from build123d import *

# Parameters (mm, degrees)
F1_DEPTH = 25.4
F0_R     = 4.1207252188
F2_DEPTH = 1.524
F4_DEPTH = 5.08
F5_R     = 4.826
F6_DEPTH = 7.62
F8_R     = 5.2675515525
F9_DEPTH = 12.7
F9_TAPER = -3


with BuildPart() as f1:
    # F0 (on Top) → F1 (new body, symmetric)
    with BuildSketch(Plane.XY):
        with BuildLine():
            ThreePointArc((1.0998522687, -0.6349999897), (1.2267258009, -0.3287001815), (1.27, 0))
            ThreePointArc((1.27, 0), (1.2267257989, 0.328700189), (1.0998522611, 0.635000003))
            ThreePointArc((1.0998522611, 0.635000003), (0.6349999985, 1.0998522637), (0, 1.27))
            ThreePointArc((0, 1.27), (-0.6349999991, 1.0998522633), (-1.0998522618, 0.6350000018))
            ThreePointArc((-1.0998522618, 0.6350000018), (-1.27, 3.4e-09), (-1.0998522652, -0.6349999959))
            ThreePointArc((-1.0998522652, -0.6349999959), (-0.6350000021, -1.0998522616), (0, -1.27))
            ThreePointArc((0, -1.27), (0.6350000051, -1.0998522598), (1.0998522687, -0.6349999897))
        make_face()
        with BuildLine():
            ThreePointArc((-1.0998522618, 0.6350000018), (-0.6349999991, 1.0998522633), (0, 1.27))
            ThreePointArc((0, 1.27), (-0.6350000007, 1.4401477376), (-1.0998522636, 1.9050000014))
            ThreePointArc((-1.0998522636, 1.9050000014), (-0.9729787264, 1.5987001881), (-0.9297045256, 1.27))
            ThreePointArc((-0.9297045256, 1.27), (-0.972978726, 0.9412998137), (-1.0998522618, 0.6350000018))
        make_face()
        with BuildLine():
            ThreePointArc((0, 1.27), (0.6349999985, 1.0998522637), (1.0998522611, 0.635000003))
            ThreePointArc((1.0998522611, 0.635000003), (0.9297045256, 1.2699999943), (1.0998522553, 1.904999987))
            ThreePointArc((1.0998522553, 1.904999987), (0.6349999935, 1.4401477334), (0, 1.27))
        make_face()
        with BuildLine():
            ThreePointArc((1.0998522611, 0.635000003), (1.2267257989, 0.328700189), (1.27, 0))
            ThreePointArc((1.27, 0), (1.2267258009, -0.3287001815), (1.0998522687, -0.6349999897))
            ThreePointArc((1.0998522687, -0.6349999897), (1.5647045337, -0.1701477325), (2.1997045323, 0))
            ThreePointArc((2.1997045323, 0), (1.564704527, 0.1701477364), (1.0998522611, 0.635000003))
        make_face()
        with BuildLine():
            ThreePointArc((1.0998522687, -1.9050000103), (0.9297045256, -1.27), (1.0998522687, -0.6349999897))
            ThreePointArc((1.0998522687, -0.6349999897), (0.6350000051, -1.0998522598), (0, -1.27))
            ThreePointArc((0, -1.27), (0.6350000051, -1.4401477402), (1.0998522687, -1.9050000103))
        make_face()
        with BuildLine():
            ThreePointArc((-1.0998522652, -1.9050000041), (-0.635000002, -1.4401477384), (0, -1.27))
            ThreePointArc((0, -1.27), (-0.6350000021, -1.0998522616), (-1.0998522652, -0.6349999959))
            ThreePointArc((-1.0998522652, -0.6349999959), (-0.9729787268, -0.9412998104), (-0.9297045256, -1.27))
            ThreePointArc((-0.9297045256, -1.27), (-0.9729787268, -1.5987001896), (-1.0998522652, -1.9050000041))
        make_face()
        with BuildLine():
            ThreePointArc((-1.0998522652, -0.6349999959), (-1.27, 3.4e-09), (-1.0998522618, 0.6350000018))
            ThreePointArc((-1.0998522618, 0.6350000018), (-1.5647045247, 0.1701477377), (-2.1997045256, 0))
            ThreePointArc((-2.1997045256, 0), (-1.5647045277, -0.170147736), (-1.0998522652, -0.6349999959))
        make_face()
        with BuildLine():
            ThreePointArc((-1.0998522636, 1.9050000014), (-0.6350000007, 1.4401477376), (0, 1.27))
            ThreePointArc((0, 1.27), (0.6349999935, 1.4401477334), (1.0998522553, 1.904999987))
            ThreePointArc((1.0998522553, 1.904999987), (1.2267257974, 2.2112998055), (1.27, 2.54))
            ThreePointArc((1.27, 2.54), (0.8980256121, 3.4380256121), (0, 3.81))
            ThreePointArc((0, 3.81), (-1.0998522624, 3.1750000007), (-1.0998522636, 1.9050000014))
        make_face()
        with BuildLine():
            ThreePointArc((-2.1997045256, 0), (-1.5647045247, 0.1701477377), (-1.0998522618, 0.6350000018))
            ThreePointArc((-1.0998522618, 0.6350000018), (-0.972978726, 0.9412998137), (-0.9297045256, 1.27))
            ThreePointArc((-0.9297045256, 1.27), (-0.9729787264, 1.5987001881), (-1.0998522636, 1.9050000014))
            ThreePointArc((-1.0998522636, 1.9050000014), (-2.1997045238, 2.54), (-3.2995567858, 1.9050000045))
            ThreePointArc((-3.2995567858, 1.9050000045), (-3.2995567897, 0.6350000022), (-2.1997045256, 0))
        make_face()
        with BuildLine():
            ThreePointArc((-0.9297045256, -1.27), (-0.9729787268, -0.9412998104), (-1.0998522652, -0.6349999959))
            ThreePointArc((-1.0998522652, -0.6349999959), (-1.5647045277, -0.170147736), (-2.1997045256, 0))
            ThreePointArc((-2.1997045256, 0), (-3.2995568097, -0.6350000369), (-3.2995567458, -1.9050000739))
            ThreePointArc((-3.2995567458, -1.9050000739), (-2.1997044853, -2.54), (-1.0998522652, -1.9050000041))
            ThreePointArc((-1.0998522652, -1.9050000041), (-0.9729787268, -1.5987001896), (-0.9297045256, -1.27))
        make_face()
        with BuildLine():
            ThreePointArc((1.0998522687, -1.9050000103), (0.6350000051, -1.4401477402), (0, -1.27))
            ThreePointArc((0, -1.27), (-0.635000002, -1.4401477384), (-1.0998522652, -1.9050000041))
            ThreePointArc((-1.0998522652, -1.9050000041), (-1.0998522616, -3.175000002), (0, -3.81))
            ThreePointArc((0, -3.81), (0.8980256121, -3.4380256121), (1.27, -2.54))
            ThreePointArc((1.27, -2.54), (1.2267258009, -2.2112998185), (1.0998522687, -1.9050000103))
        make_face()
        with BuildLine():
            ThreePointArc((2.1997045323, 0), (1.5647045337, -0.1701477325), (1.0998522687, -0.6349999897))
            ThreePointArc((1.0998522687, -0.6349999897), (0.9297045256, -1.27), (1.0998522687, -1.9050000103))
            ThreePointArc((1.0998522687, -1.9050000103), (2.1997045101, -2.54), (3.299556767, -1.9050000371))
            ThreePointArc((3.299556767, -1.9050000371), (3.4264303195, -1.598700208), (3.4697045256, -1.27))
            ThreePointArc((3.4697045256, -1.27), (3.0977301401, -0.3719743903), (2.1997045323, 0))
        make_face()
        with BuildLine():
            ThreePointArc((1.0998522553, 1.904999987), (0.9297045256, 1.2699999943), (1.0998522611, 0.635000003))
            ThreePointArc((1.0998522611, 0.635000003), (1.564704527, 0.1701477364), (2.1997045323, 0))
            ThreePointArc((2.1997045323, 0), (3.0977301401, 0.3719743903), (3.4697045256, 1.27))
            ThreePointArc((3.4697045256, 1.27), (3.4264303195, 1.598700208), (3.299556767, 1.9050000371))
            ThreePointArc((3.299556767, 1.9050000371), (2.1997044967, 2.54), (1.0998522553, 1.904999987))
        make_face()
    extrude(amount=F1_DEPTH, both=True)

    # F0 (on Top) → F2 (join, symmetric)
    with BuildSketch(Plane.XY):
        Circle(F0_R)
        with BuildLine():
            ThreePointArc((0, 3.81), (1.9049999814, 3.2995567991), (3.299556767, 1.9050000371))
            ThreePointArc((3.299556767, 1.9050000371), (3.6801773926, 0.9861005825), (3.81, 0))
            ThreePointArc((3.81, 0), (3.6801773926, -0.9861005825), (3.299556767, -1.9050000371))
            ThreePointArc((3.299556767, -1.9050000371), (1.9049999814, -3.2995567991), (0, -3.81))
            ThreePointArc((0, -3.81), (-1.9049999631, -3.2995568097), (-3.2995567458, -1.9050000739))
            ThreePointArc((-3.2995567458, -1.9050000739), (-3.81, -4.01e-08), (-3.2995567858, 1.9050000045))
            ThreePointArc((-3.2995567858, 1.9050000045), (-1.9049999978, 3.2995567897), (0, 3.81))
        make_face(mode=Mode.SUBTRACT)
        with BuildLine():
            ThreePointArc((-3.2995567858, 1.9050000045), (-2.1997045238, 2.54), (-1.0998522636, 1.9050000014))
            ThreePointArc((-1.0998522636, 1.9050000014), (-1.0998522624, 3.1750000007), (0, 3.81))
            ThreePointArc((0, 3.81), (-1.9049999978, 3.2995567897), (-3.2995567858, 1.9050000045))
        make_face()
        with BuildLine():
            ThreePointArc((1.27, 2.54), (1.2267257974, 2.2112998055), (1.0998522553, 1.904999987))
            ThreePointArc((1.0998522553, 1.904999987), (2.1997044967, 2.54), (3.299556767, 1.9050000371))
            ThreePointArc((3.299556767, 1.9050000371), (1.9049999814, 3.2995567991), (0, 3.81))
            ThreePointArc((0, 3.81), (0.8980256121, 3.4380256121), (1.27, 2.54))
        make_face()
        with BuildLine():
            ThreePointArc((3.4697045256, 1.27), (3.0977301401, 0.3719743903), (2.1997045323, 0))
            ThreePointArc((2.1997045323, 0), (3.0977301401, -0.3719743903), (3.4697045256, -1.27))
            ThreePointArc((3.4697045256, -1.27), (3.4264303195, -1.598700208), (3.299556767, -1.9050000371))
            ThreePointArc((3.299556767, -1.9050000371), (3.6801773926, -0.9861005825), (3.81, 0))
            ThreePointArc((3.81, 0), (3.6801773926, 0.9861005825), (3.299556767, 1.9050000371))
            ThreePointArc((3.299556767, 1.9050000371), (3.4264303195, 1.598700208), (3.4697045256, 1.27))
        make_face()
        with BuildLine():
            ThreePointArc((3.299556767, -1.9050000371), (2.1997045101, -2.54), (1.0998522687, -1.9050000103))
            ThreePointArc((1.0998522687, -1.9050000103), (1.2267258009, -2.2112998185), (1.27, -2.54))
            ThreePointArc((1.27, -2.54), (0.8980256121, -3.4380256121), (0, -3.81))
            ThreePointArc((0, -3.81), (1.9049999814, -3.2995567991), (3.299556767, -1.9050000371))
        make_face()
        with BuildLine():
            ThreePointArc((0, -3.81), (-1.0998522616, -3.175000002), (-1.0998522652, -1.9050000041))
            ThreePointArc((-1.0998522652, -1.9050000041), (-2.1997044853, -2.54), (-3.2995567458, -1.9050000739))
            ThreePointArc((-3.2995567458, -1.9050000739), (-1.9049999631, -3.2995568097), (0, -3.81))
        make_face()
        with BuildLine():
            ThreePointArc((-3.2995567458, -1.9050000739), (-3.2995568097, -0.6350000369), (-2.1997045256, 0))
            ThreePointArc((-2.1997045256, 0), (-3.2995567897, 0.6350000022), (-3.2995567858, 1.9050000045))
            ThreePointArc((-3.2995567858, 1.9050000045), (-3.81, -4.01e-08), (-3.2995567458, -1.9050000739))
        make_face()
    extrude(amount=F2_DEPTH, both=True)

    # F3 (on face) → F4 (cut)
    with BuildSketch(Plane.XY.offset(25.4)):
        with BuildLine():
            ThreePointArc((1.1617240994, -0.5382236443), (1.2503393833, -0.2755703193), (1.2803466618, 0))
            ThreePointArc((1.2803466618, 0), (1.2503393833, 0.2755703193), (1.1617240994, 0.5382236443))
            ThreePointArc((1.1617240994, 0.5382236443), (1.0998522628, 0.635), (1.0469773986, 0.7369707601))
            ThreePointArc((1.0469773986, 0.7369707601), (0.6401733309, 1.1088127348), (0.1147467008, 1.2751944044))
            ThreePointArc((0.1147467008, 1.2751944044), (0, 1.27), (-0.1147467008, 1.2751944044))
            ThreePointArc((-0.1147467008, 1.2751944044), (-0.6401733309, 1.1088127348), (-1.0469773986, 0.7369707601))
            ThreePointArc((-1.0469773986, 0.7369707601), (-1.0998522628, 0.635), (-1.1617240994, 0.5382236443))
            ThreePointArc((-1.1617240994, 0.5382236443), (-1.2803466618, 0), (-1.1617240994, -0.5382236443))
            ThreePointArc((-1.1617240994, -0.5382236443), (-1.0998522628, -0.635), (-1.0469773986, -0.7369707601))
            ThreePointArc((-1.0469773986, -0.7369707601), (-0.6401733309, -1.1088127348), (-0.1147467008, -1.2751944044))
            ThreePointArc((-0.1147467008, -1.2751944044), (0, -1.27), (0.1147467008, -1.2751944044))
            ThreePointArc((0.1147467008, -1.2751944044), (0.6401733309, -1.1088127348), (1.0469773986, -0.7369707601))
            ThreePointArc((1.0469773986, -0.7369707601), (1.0998522628, -0.635), (1.1617240994, -0.5382236443))
        make_face()
    extrude(amount=-F4_DEPTH, mode=Mode.SUBTRACT)

    # F5 (on face) → F6 (join)
    with BuildSketch(Plane.XY.offset(25.4)):
        Circle(F5_R)
        with BuildLine():
            ThreePointArc((0.4317572455, 3.7343557598), (2.8066798027, 2.5008749959), (3.75923227, 0))
            ThreePointArc((3.75923227, 0), (-2.5008749959, -2.8066798027), (-0.4317572455, 3.7343557598))
            ThreePointArc((-0.4317572455, 3.7343557598), (0, 3.81), (0.4317572455, 3.7343557598))
        make_face(mode=Mode.SUBTRACT)
    extrude(amount=-F6_DEPTH)

    # F8 (on offset) → F9 (join)
    with BuildSketch(Plane(origin=(0, 0, -25.4), x_dir=(1, 0, 0), z_dir=(0, 0, -1))):
        Circle(F8_R)
    extrude(amount=F9_DEPTH, taper=F9_TAPER)


solid = f1.part
Part model, mm, in its own coordinate system. A direction names the side the tool comes from. Give positions to 0.01 mm unless a question says otherwise; leave off trailing zeros. Write each loop counter-clockwise with the first axis right and the second up, starting at its lowest first coordinate (ties: lowest second). Pieces come first, ordered by that corner, then holes.
1) Two-plate mould, pull along X, no slides. Class faces 1 (the face through (5.346, -1.684, -31.839)), 2 (the face through (0, -4, 17.78)), 3 (the face through (-3.76, -0.02, 21.64)): released by +X, released by -X, zero draft, split by the parting line, or undercut.
Resolved:
face 1: split by the parting line
face 2: zero draft
face 3: undercut
2) Pin check, flat tips, straight feed: pin 1 (4 mm diameter, centred on x = -4.5, z = -31, fed in from -Y); pin 2 (3 mm diameter, centred on x = -3.5, z = 10.5, fed in from +Y); pin 3 (1.5 mm diameter, centred on x = 3.5, z = -3.5, fed in from +Y). Stop position of each tip, or through.
Resolved:
pin 1: stops at y = -4.97
pin 2: stops at y = 2.54
pin 3: stops at y = 2.41
3) Cut at A-A on z = -5. Write the cut outline in (x, y) (3 decimals).
Resolved:
outline: (-2.2, 0) arc R1.27 ccw (long way) to (-1.1, -1.905) arc R1.27 ccw (long way) to (1.1, -1.905) arc R1.27 ccw (long way) to (2.2, 0) arc R1.27 ccw (long way) to (1.1, 1.905) arc R1.27 ccw (long way) to (-1.1, 1.905) arc R1.27 ccw (long way) to start
4) Probe L1, parallel to Z at x = -2.25, y = 3.25; L2, parallel to Z at x = 1.5, y = -4; L3, parallel to Z at x = 1, y = 3.5. List the from-to ranges inside material, lowest first.
Resolved:
L1: z = -38.1 to -25.4, -1.52 to 1.52, 17.78 to 25.4
L2: z = -38.1 to -25.4, 17.78 to 25.4
L3: z = -38.1 to -25.4, -1.52 to 1.52
5) Which spindle directions (+Z, -Z, +X, -X, +Y, -Y) get a long thin tool onto all of the face, cutting with end or side? Do faces 4 (the face through (3, 0, 1.524)), 5 (the face through (0, 0, -38.1)), 6 (the face through (0, 0, 20.32)). Say none if no direction does.
Resolved:
face 4: none
face 5: -Z, +X, -X, +Y, -Y
face 6: +Z
